```python
from build123d import *

# Parameters (mm, degrees)
SKETCH1_W           = 6.35
SKETCH1_H           = 6.35
BOSS_EXTRUDE1_DEPTH = 94.45625
SKETCH2_W           = 7.9375
SKETCH2_H           = 7.9375
SKETCH2_R           = 3.175
CUT_EXTRUDE1_DEPTH  = 3.175
CUT_EXTRUDE2_DEPTH  = 42.8625


with BuildPart() as part:
    # Sketch1 → Boss-Extrude1 (new body)
    with BuildSketch(Plane(origin=(0, 0, 0), x_dir=(0, 0, -1), z_dir=(1, 0, 0))):
        Rectangle(SKETCH1_W, SKETCH1_H)
    extrude(amount=BOSS_EXTRUDE1_DEPTH)

    # Sketch2 → Cut-Extrude1 (cut)
    with BuildSketch(Plane(origin=(94.45625, 0, 0), x_dir=(0, 0, -1), z_dir=(1, 0, 0))):
        Rectangle(SKETCH2_W, SKETCH2_H)
        Circle(SKETCH2_R, mode=Mode.SUBTRACT)
    extrude(amount=-CUT_EXTRUDE1_DEPTH, mode=Mode.SUBTRACT)

    # Sketch3 → Cut-Extrude2 (cut)
    with BuildSketch(Plane(origin=(91.28125, 0, 0), x_dir=(0, 0, -1), z_dir=(1, 0, 0))):
        with BuildLine():
            Line((-3.175, -2.432976572), (-3.175, -3.175))
            Line((-3.175, -3.175), (-2.432976572, -3.175))
            ThreePointArc((-2.432976572, -3.175), (-2.828427125, -2.828427125), (-3.175, -2.432976572))
        make_face()
        with BuildLine():
            Line((2.432976572, -3.175), (3.175, -3.175))
            Line((3.175, -3.175), (3.175, -2.432976572))
            ThreePointArc((3.175, -2.432976572), (2.828427125, -2.828427125), (2.432976572, -3.175))
        make_face()
        with BuildLine():
            Line((3.175, 2.432976572), (3.175, 3.175))
            Line((3.175, 3.175), (2.432976572, 3.175))
            ThreePointArc((2.432976572, 3.175), (2.828427125, 2.828427125), (3.175, 2.432976572))
        make_face()
        with BuildLine():
            Line((-3.175, 3.175), (-3.175, 2.432976572))
            ThreePointArc((-3.175, 2.432976572), (-2.828427125, 2.828427125), (-2.432976572, 3.175))
            Line((-2.432976572, 3.175), (-3.175, 3.175))
        make_face()
    extrude(amount=-CUT_EXTRUDE2_DEPTH, mode=Mode.SUBTRACT)

    # Mirror1: part across plane


with BuildPart() as part_1:
    add(part.part)
    add(part.part.mirror(Plane(origin=(0, 0, 0), x_dir=(0, 0, 1), z_dir=(1, 0, 0))))


solid = part_1.part
```
Geometry: final body of the model. Coordinates: model frame, mm. A direction names the side the tool comes from. Round coordinates to 2 decimals unless told otherwise and drop trailing zeros. Order: outer loops, then holes, each group sorted by start corner. A loop starts at its lowest first (then second) coordinate and runs counter-clockwise, first axis right, second up. Notation, with made-up numbers: (38.5, -14) -> (97.5, -14) arc R26 ccw to (97.5, 23) -> close; hole circle Ø4 at (78.25, 19.25). An arc over 180 degrees is marked (long way). Use one line per item in the form item = value.
(1) First-contact query: pin 1 Ø0.8 at (y, z) = (-3, 3) entering from -X; pin 2 Ø0.8 at (y, z) = (-3, -3) entering from +X. Flat tips, straight axial feed; report the tip coordinate or a pass-through.
Results list:
pin_1 = -91.28
pin_2 = 91.28
(2) Access query for faces 1 (the face through (-91.281, 3, -2)), 2 (the face through (91.281, -2.4, 2.4)), 3 (the face through (-91.281, 2.3, 2.42)), 4 (the face through (92.89, -3.1, 0.69)). Directions: +Z, -Z, +X, -X, +Y, -Y. A direction counts if a zero-diameter tool reaches every point of the face in a straight line with its end or side. Return the directions, or none.
Results list:
face_1 = -Z, -X, +Y
face_2 = +Z, +X, -Y
face_3 = +Z, -X, +Y
face_4 = +X
(3) Section A-A on x = -52. Return loops of the section in (y, z) (3 decimals), and give its area (3 significant figures).
Results list:
outline = (-3.175, -2.433) arc R4 ccw to (-2.433, -3.175) -> (2.433, -3.175) arc R4 ccw to (3.175, -2.433) -> (3.175, 2.433) arc R4 ccw to (2.433, 3.175) -> (-2.433, 3.175) arc R4 ccw to (-3.175, 2.433) -> close
area = 39.3 mm^2
(4) Ray query, probe 1 along Y at (x, z) = (-73, -3); probe 2 along Z at (x, y) = (48.5, 2.75); probe 3 along Z at (x, y) = (-55, -2.5). Return the intervals inside material, ascending. Write a range as [from, to].
Results list:
probe_1 = [-2.65, 2.65]
probe_2 = [-2.9, 2.9]
probe_3 = [-3.12, 3.12]
